Verification items for the finished model (mm, model axes). Coordinates: 2 decimals unless noted, no trailing zeros. Write each loop counter-clockwise with the first axis right and the second up, starting at its lowest first coordinate (ties: lowest second). Pieces come first, ordered by that corner, then holes. Notation, with made-up numbers: (-8.5, -7) -> (11.5, -7) arc R12 cw to (11.5, 9) -> close; hole circle Ø10 at (17, 30). An arc over 180 degrees is marked (long way). Answer in a Markdown table with one row per item.
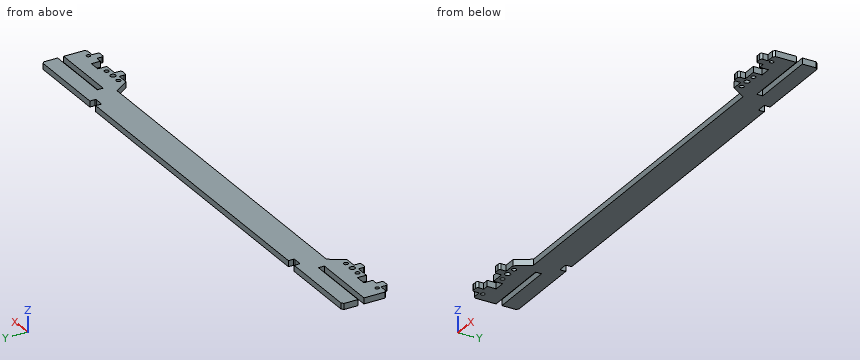
Autodesk Inventor part; units mm, degrees
ref_plane "YZ Plane" through (0, 0, 0) normal (1, 0, 0) x (0, 1, 0)
ref_plane "XZ Plane" through (0, 0, 0) normal (0, 1, 0) x (-1, 0, 0)
ref_plane "XY Plane" through (0, 0, 0) normal (0, 0, 1) x (1, 0, 0)
sketch "Sketch1" plane through (0, 0, 0) normal (0, 0, 1) x (1, 0, 0)
  line L0 (516, 45) -> (0, 45)
  line L1 (68, 0) -> (78, 15)
  line L2 (78, 15) -> (438, 15)
  line L3 (438, 15) -> (448, 0)
  line L4 (0, 0) -> (68, 0)
  line L5 (448, 0) -> (516, 0)
  line L6 (0, 29) -> (68, 29)
  line L7 (68, 29) -> (68, 23)
  line L8 (68, 23) -> (0, 23)
  line L9 (0, 45) -> (0, 29)
  line L10 (0, 23) -> (0, 0)
  line L11 (516, 29) -> (448, 29)
  line L12 (448, 29) -> (448, 23)
  line L13 (448, 23) -> (516, 23)
  line L14 (516, 0) -> (516, 23)
  line L15 (516, 29) -> (516, 45)
  dimension "d3" = 6
  dimension "d4" = 68
  dimension "d5" = 68
  dimension "d6" = 516
  dimension "d7" = 15
  dimension "d8" = 23
  dimension "d9" = 16
  dimension "d12" = 10
  dimension "d13" = 10
  dimension "d14" = 10
  dimension "d15" = 10
extrude "Extrusion1" add sketch "Sketch1" along normal blind 6
sketch "Sketch2" plane through (0, 0, 6) normal (0, 0, 1) x (1, 0, 0)
  line L0 (0, 0) -> (68, 0)
  line L1 (448, 0) -> (516, 0)
  line L2 (516, 0) -> (516, 23)
  line L3 (516, 29) -> (516, 45)
  line L4 (516, 45) -> (0, 45)
  line L5 (0, 45) -> (0, 29)
  line L6 (0, 23) -> (0, 0)
  line L7 (24, 0) -> (35, 0)
  line L8 (35, 0) -> (35, 9)
  line L9 (35, 9) -> (24, 9)
  line L10 (24, 9) -> (24, 0)
  circle A0 centre (42.5, 4.5) radius 2.25
  circle A1 centre (52.5, 3.901) radius 2.75
  circle A2 centre (62.5, 4.5) radius 2.25
  line L11 (492, 0) -> (481, 0)
  line L12 (481, 0) -> (481, 9)
  line L13 (481, 9) -> (492, 9)
  line L14 (492, 9) -> (492, 0)
  circle A3 centre (453.5, 4.5) radius 2.25
  circle A4 centre (463.5, 3.901) radius 2.75
  circle A5 centre (473.5, 4.5) radius 2.25
  line L15 (82.5, 45) -> (92.5, 45)
  line L16 (92.5, 45) -> (92.5, 40)
  line L17 (91.5, 39) -> (83.5, 39)
  line L18 (82.5, 40) -> (82.5, 45)
  line L19 (423.5, 45) -> (433.5, 45)
  line L20 (433.5, 45) -> (433.5, 40)
  line L21 (432.5, 39) -> (424.5, 39)
  line L22 (423.5, 40) -> (423.5, 45)
  arc A6 (82.5, 40) -> (83.5, 39) centre (83.5, 40) ccw
  arc A7 (91.5, 39) -> (92.5, 40) centre (91.5, 40) ccw
  arc A8 (423.5, 40) -> (424.5, 39) centre (424.5, 40) ccw
  arc A9 (432.5, 39) -> (433.5, 40) centre (432.5, 40) ccw
  circle A10 centre (29.5, 3.901) radius 7.5 construction
  point P0 (486.5, 9)
  point P1 (35, 4.5)
  point P2 (87.5, 39)
  point P3 (428.5, 39)
  dimension "d16" = 11
  dimension "d18" = 4.5
  dimension "d19" = 5.5
  dimension "d20" = 11
  dimension "d21" = 1
  dimension "d22" = 10
  dimension "d23" = 10
  dimension "d24" = 6
  dimension "d27" = 24
  dimension "d29" = 23
  dimension "d30" = 24
  dimension "d31" = 10
  dimension "d32" = 10
  dimension "d33" = 10
  dimension "d34" = 10
  dimension "d35" = 9
  dimension "d38" = 15
  dimension "d39" = 23
  dimension "d49" = 87.5
  dimension "d50" = 87.5
extrude "Extrusion2" cut sketch "Sketch2" against normal blind 6
chamfer "Chamfer1" distance 2 angle 45 4 edges at (0, 45, 3) (0, 0, 3) (516, 45, 3) (516, 0, 3)
sketch "Sketch3" plane through (0, 0, 6) normal (0, 0, 1) x (1, 0, 0)
  line L0 (516, 2) -> (516, 23)
  line L1 (0, 23) -> (0, 2)
  circle A0 centre (52.5, 3.901) radius 2.75
  circle A1 centre (10, 3.901) radius 2
  circle A2 centre (506, 3.901) radius 2
  point P0 (0, 0)
  dimension "d43" = 4
  dimension "d44" = 10
  dimension "d45" = 4
  dimension "d46" = 10
extrude "Extrusion3" cut sketch "Sketch3" against normal through all contours A1 | A2
sketch "Sketch4" plane through (0, 0, 6) normal (0, 0, 1) x (1, 0, 0)
  line L0 (516, 2) -> (516, 23)
  line L1 (0, 23) -> (0, 2)
  line L2 (2, 0) -> (24, 0)
  line L3 (35, 0) -> (68, 0)
  line L4 (448, 0) -> (481, 0)
  line L5 (492, 0) -> (514, 0)
  line L6 (10, 0) -> (18, 0)
  line L7 (18, 0) -> (18, -5)
  line L8 (16, -7) -> (12, -7)
  line L9 (10, -5) -> (10, 0)
  line L10 (48.5, 0) -> (56.5, 0)
  line L11 (56.5, 0) -> (56.5, -5)
  line L12 (54.5, -7) -> (50.5, -7)
  line L13 (48.5, -5) -> (48.5, 0)
  line L14 (459.5, 0) -> (467.5, 0)
  line L15 (467.5, 0) -> (467.5, -5)
  line L16 (465.5, -7) -> (461.5, -7)
  line L17 (459.5, -5) -> (459.5, 0)
  line L18 (498, 0) -> (506, 0)
  line L19 (506, 0) -> (506, -5)
  line L20 (504, -7) -> (500, -7)
  line L21 (498, -5) -> (498, 0)
  arc A0 (10, -5) -> (12, -7) centre (12, -5) ccw
  arc A1 (16, -7) -> (18, -5) centre (16, -5) ccw
  arc A2 (48.5, -5) -> (50.5, -7) centre (50.5, -5) ccw
  arc A3 (54.5, -7) -> (56.5, -5) centre (54.5, -5) ccw
  arc A4 (459.5, -5) -> (461.5, -7) centre (461.5, -5) ccw
  arc A5 (465.5, -7) -> (467.5, -5) centre (465.5, -5) ccw
  arc A6 (498, -5) -> (500, -7) centre (500, -5) ccw
  arc A7 (504, -7) -> (506, -5) centre (504, -5) ccw
  point P0 (0, 0)
  dimension "d51" = 2
  dimension "d52" = 8
  dimension "d53" = 8
  dimension "d54" = 8
  dimension "d55" = 8
  dimension "d56" = 7
  dimension "d57" = 10
  dimension "d58" = 30.5
  dimension "d59" = 10
  dimension "d60" = 30.5
extrude "Extrusion4" add sketch "Sketch4" against normal blind 6
equation "\"d5\" = d4"
equation "\"d20\" = d16"
equation "\"d23\" = d22"
equation "\"d30\" = d27"
equation "\"d45\" = d43"
equation "\"d46\" = d44"
equation "\"d59\" = d57"
equation "\"d60\" = d58"
properties part number "x_axis_chain_holder"
1. Sectioned sample at B-B, the plane z = 1.8. Count the separate pieces of the cut face and the enclosed holes in it, and give its area (3 significant figures).
Findings below:
| item | result |
|---|---|
| separate pieces | 1 |
| enclosed holes | 8 |
| area | 16,600 mm² |
2. Sectioned sample at A-A, the plane x = 152. Record the cut outline in (y, z).
Findings below:
| item | result |
|---|---|
| outline | (15, 0) -> (45, 0) -> (45, 6) -> (15, 6) -> close |
3. Go/stop test with flat-tipped pins: pin 1 (12 mm diameter, centred on x = 208.5, y = 5.5, fed in from -Z); pin 2 (1 mm diameter, centred on x = 396.5, y = 19, fed in from -Z); pin 3 (2.5 mm diameter, centred on y = -2.5, z = 4.5, fed in from -X); pin 4 (1.8 mm diameter, centred on x = 495.5, z = 4.5, fed in from -Y). Record where each tip stops, or that it passes through.
Findings below:
| item | result |
|---|---|
| pin 1 | passes through |
| pin 2 | stops at z = 0 |
| pin 3 | stops at x = 10 |
| pin 4 | stops at y = 0 |
4. Material ranges on probe 1 along X at (y, z) = (-2.5, 1); probe 2 along Y at (x, z) = (52.5, 2.05); probe 3 along Y at (x, z) = (42.5, 3.5), recorded low to high. Write a range as from..to.
Findings below:
| item | result |
|---|---|
| probe 1 | x = 10..18, 48.5..56.5, 459.5..467.5, 498..506 |
| probe 2 | y = -7..1.15, 6.65..23, 29..45 |
| probe 3 | y = 0..2.25, 6.75..23, 29..45 |
